```python
from build123d import *

# Parameters (mm, degrees)
SKETCH_R     = 0.75
PAD_DEPTH    = 1
SKETCH001_R  = 1.5
PAD001_DEPTH = 2
PAD002_DEPTH = 2
SKETCH003_R  = 0.45
PAD003_DEPTH = 3.75


with BuildPart() as part:
    # Sketch → Pad (new body)
    with BuildSketch(Plane.XY):
        with BuildLine():
            ThreePointArc((10.84, -2.1), (12.94, 0), (10.84, 2.1))
            Line((10.84, 2.1), (-10.84, 2.1))
            ThreePointArc((-10.84, 2.1), (-12.94, 0), (-10.84, -2.1))
            Line((10.84, -2.1), (-10.84, -2.1))
        make_face()
        with Locations((-11.49, 0)):
            Circle(SKETCH_R, mode=Mode.SUBTRACT)
        with Locations((11.49, 0)):
            Circle(SKETCH_R, mode=Mode.SUBTRACT)
    extrude(amount=-PAD_DEPTH)

    # Sketch001 → Pad001 (join)
    with BuildSketch(Plane.XY):
        with BuildLine():
            ThreePointArc((-7.94, 2.1), (-10.04, 0), (-7.94, -2.1))
            Line((-7.94, -2.1), (7.94, -2.1))
            ThreePointArc((7.94, -2.1), (10.04, 0), (7.94, 2.1))
            Line((-7.94, 2.1), (7.94, 2.1))
        make_face()
        with Locations((-7.94, 0)):
            Circle(SKETCH001_R, mode=Mode.SUBTRACT)
        with Locations((7.94, 0)):
            Circle(SKETCH001_R, mode=Mode.SUBTRACT)
    extrude(amount=PAD001_DEPTH)

    # Sketch002 → Pad002 (join)
    with BuildSketch(Plane.XY):
        with BuildLine():
            ThreePointArc((-7.939999, 2.1), (-10.039999, 0), (-7.939999, -2.1))
            Line((-7.939999, -2.1), (7.94, -2.1))
            ThreePointArc((7.94, -2.1), (10.04, 0), (7.94, 2.1))
            Line((-7.939999, 2.1), (7.94, 2.1))
        make_face()
    extrude(amount=-PAD002_DEPTH)

    # Sketch003 → Pad003 (join)
    with BuildSketch(Plane.XY):
        with Locations((-5.08, 0)):
            Circle(SKETCH003_R)
        with Locations((-2.54, 0)):
            Circle(SKETCH003_R)
        Circle(SKETCH003_R)
        with Locations((2.54, 0)):
            Circle(SKETCH003_R)
        with Locations((5.08, 0)):
            Circle(SKETCH003_R)
    extrude(amount=-PAD003_DEPTH)


solid = part.part
```
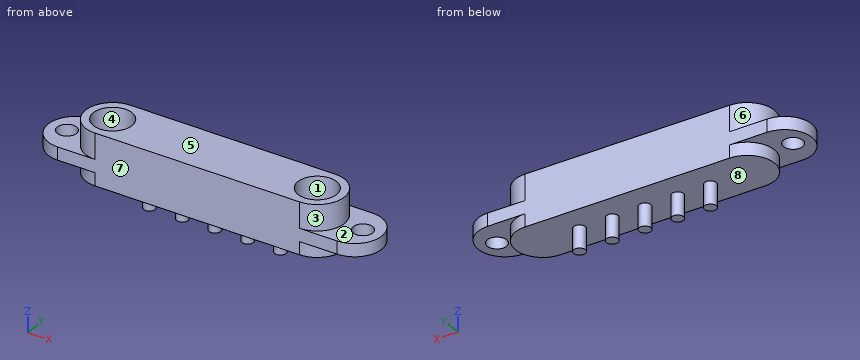
The model under review builds one solid part; all positions refer to its coordinate system, in mm. Face numbers are marked on the shaded views. A direction names the side the tool comes from. Give positions to 0.01 mm unless a question says otherwise; leave off trailing zeros. Write each loop counter-clockwise with the first axis right and the second up, starting at its lowest first coordinate (ties: lowest second). Pieces come first, ordered by that corner, then holes.
(1) Consider section C-C, the plane x = 0. Give the boundary of the cut face in (y, z), and give its area (3 significant figures).
(2) To check wall thickness, follow L1, parallel to Y at x = 7.94, z = 0.5; L2, parallel to Y at x = -11.49, z = -0.15; L3, parallel to Z at x = 3.5, y = -1.5. State the ranges of each line that lie inside material, in increasing order.
(3) Consider section D-D, the plane y = 0. Give the number of separate pieces and of enclosed holes in the cut face, and give its area (3 significant figures).
(4) For P1, Ø2.5, axis at x = -7.94, y = 0, coming from the +Z side; P2, Ø1.3, axis at x = 10, y = -0.5, coming from the +Z side, all flat-tipped, find the tip position at first contact; note any pin that passes through.
(5) Tool access review of the marked faces 4, 5, 6, 7 and 8: name each direction out of +Z, -Z, +X, -X, +Y, -Y from which nothing blocks a thin tool from reaching the whole face with its end or side.
(6) Consider section A-A, the plane z = -2.5. Give the boundary of the cut face in (x, y).
(7) The part is to be moulded in two halves that separate along Y. For the marked faces 1, 2 and 3, say which applies: released by +Y, released by -Y, zero draft, split by the parting line, or undercut.
(8) Consider section B-B, the plane z = 1.05. Give the boundary of the cut face in (x, y).
Returned:
1. outline: (-2.1, -2) - (-0.45, -2) - (-0.45, -3.75) - (0.45, -3.75) - (0.45, -2) - (2.1, -2) - (2.1, 2) - (-2.1, 2) - close
1. area: 18.4 mm2
2. L1: y = -2.1 to -1.5, 1.5 to 2.1
2. L2: y = -2 to -0.75, 0.75 to 2
2. L3: z = -2 to 2
3. separate pieces: 3
3. enclosed holes: 0
3. area: 79.0 mm2
4. P1: stops at z = 0
4. P2: stops at z = 2
5. face 4: +Z
5. face 5: +Z, +X, -X, +Y, -Y
5. face 6: +Z, -X
5. face 7: +Z, -Z, +X, -X, -Y
5. face 8: -Z
6. outline: circle Ø0.9 at (-5.08, 0); circle Ø0.9 at (-2.54, 0); circle Ø0.9 at (0, 0); circle Ø0.9 at (2.54, 0); circle Ø0.9 at (5.08, 0)
7. face 1: undercut
7. face 2: zero draft
7. face 3: split by the parting line
8. outline: (-7.94, -2.1) - (7.94, -2.1) arc R2.1 ccw to (7.94, 2.1) - (-7.94, 2.1) arc R2.1 ccw to start; hole circle Ø3 at (-7.94, 0); hole circle Ø3 at (7.94, 0)
